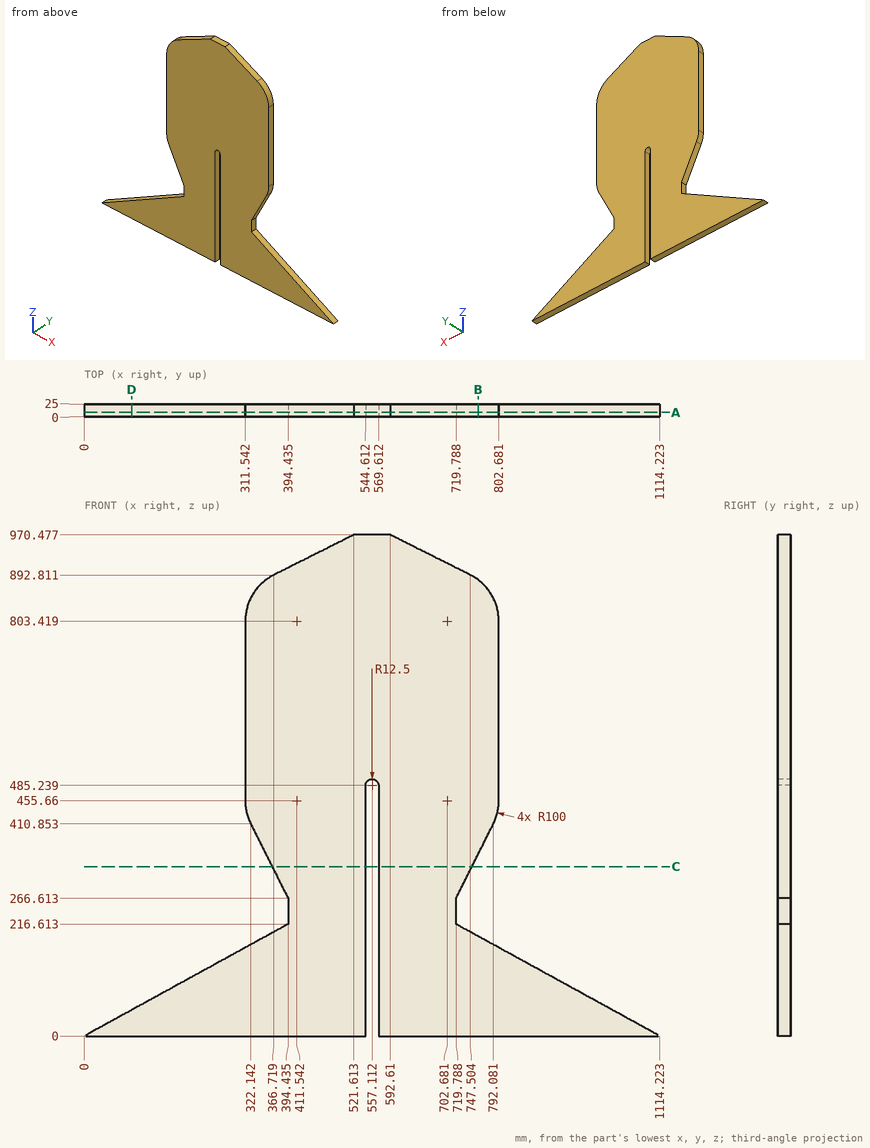
Source: three-view drawing plus pictorial views. Frame: mm from the lowest corner of the part. Give positions to 0.01 mm unless a question says otherwise; leave off trailing zeros. Write each loop counter-clockwise with the first axis right and the second up, starting at its lowest first coordinate (ties: lowest second). Pieces come first, ordered by that corner, then holes.
(1) Cut plane C-C, the plane z = 328. Return loops of the section in (x, y) (1 decimal), then the cut area to 3 significant figures.
(2) Ray query, line 1 (X direction, y = 17, z = 779.5); line 2 (Z direction, x = 730, y = 5.5) (1 decimal); line 3 (X direction, y = 5.5, z = 256.5) (1 decimal). Return the intervals inside material, ascending.
(3) First-contact query: P1, Ø12.5, axis at y = 6.5, z = 233.5, coming from the +X side; P2, Ø5, axis at x = 952.5, y = 15.5, coming from the +Z side; P3, Ø4, axis at y = 3.5, z = 592.5, coming from the +X side. Flat tips, straight axial feed; report the tip coordinate or a pass-through.
(4) Cut plane A-A, the plane y = 9. Return loops of the section in (x, z) (1 decimal), then the cut area to 3 significant figures.
(5) Cut plane D-D, the plane x = 91.5. Return loops of the section in (y, z), then the cut area to 3 significant figures.
(6) Cut plane B-B, the plane x = 762.5. Return loops of the section in (y, z) (1 decimal), then the cut area to 3 significant figures.
Values follow:
1. outline: (363.7, 0) - (544.6, 0) - (544.6, 25) - (363.7, 25) - close; (569.6, 0) - (750.6, 0) - (750.6, 25) - (569.6, 25) - close
1. area: 9,050 mm2
2. line 1: x = 311.54 to 802.68
2. line 2: z = 0 to 211, 287 to 901.6
2. line 3: x = 394.4 to 544.6, 569.6 to 719.8
3. P1: stops at x = 719.79
3. P2: stops at z = 90.19
3. P3: stops at x = 802.68
4. outline: (0, 0) - (544.6, 0) - (544.6, 485.3) arc R12.5 cw to (569.6, 485.3) - (569.6, 0) - (1114.2, 0) - (719.8, 216.6) - (719.8, 266.6) - (792.1, 410.9) arc R100 ccw to (802.7, 455.7) - (802.7, 803.4) arc R100 ccw to (747.5, 892.8) - (592.6, 970.5) - (521.6, 970.5) - (366.7, 892.8) arc R100 ccw to (311.5, 803.4) - (311.5, 455.7) arc R100 ccw to (322.1, 410.9) - (394.4, 266.6) - (394.4, 216.6) - close
4. area: 468,000 mm2
5. outline: (0, 0) - (25, 0) - (25, 50.25) - (0, 50.25) - close
5. area: 1,260 mm2
6. outline: (0, 0) - (25, 0) - (25, 193.2) - (0, 193.2) - close; (0, 351.8) - (25, 351.8) - (25, 883.6) - (0, 883.6) - close
6. area: 18,100 mm2
